```python
from build123d import *

# Parameters (mm, degrees)
SKETCH_1_R               = 4
EXTRUDE_1_DEPTH          = 5.5
SKETCH_2_R               = 1.2
EXTRUDE_2_DEPTH          = 11
SKETCH_6_R               = 0.75
CUT_EXTRUDE_1_DEPTH      = 5
CUT_EXTRUDE_1_DEPTH_BACK = 5
SKETCH_7_R               = 4
CUT_EXTRUDE_2_DEPTH      = 1


with BuildPart() as part:
    # ｽｹｯﾁ1 → ﾎﾞｽ - 押し出し1 (new body)
    with BuildSketch(Plane.XY):
        Circle(SKETCH_1_R)
    extrude(amount=EXTRUDE_1_DEPTH)

    # ｽｹｯﾁ2 → ﾎﾞｽ - 押し出し2 (add)
    with BuildSketch(Plane.XY.offset(5.5)):
        Circle(SKETCH_2_R)
    extrude(amount=EXTRUDE_2_DEPTH)

    # ｽｹｯﾁ4 → ｶｯﾄ - 回転1 (revolve, cut)
    with BuildSketch(Plane(origin=(0, 0, 0), x_dir=(1, 0, 0), z_dir=(0, 1, 0))):
        Polygon((1.2, -16.5), (0.711175277, -16.5), (1.15, -15.5), (0.95, -13.2), (1.2, -12.7), align=None)
    revolve(axis=Axis((0, 0, 12.792952675), (0, 0, 1)), mode=Mode.SUBTRACT)

    # ｽｹｯﾁ6 → ｶｯﾄ - 押し出し1 (cut, two sides)
    with BuildSketch(Plane(origin=(0, 0, 0), x_dir=(1, 0, 0), z_dir=(0, 1, 0))) as cut_extrude_1_sk:
        with Locations((0, -3)):
            Circle(SKETCH_6_R)
    extrude(amount=CUT_EXTRUDE_1_DEPTH, mode=Mode.SUBTRACT)
    extrude(cut_extrude_1_sk.sketch, amount=-CUT_EXTRUDE_1_DEPTH_BACK, mode=Mode.SUBTRACT)

    # ｽｹｯﾁ7 → ｶｯﾄ - 押し出し2 (cut)
    with BuildSketch(Plane(origin=(0, 0, 0), x_dir=(-1, 0, 0), z_dir=(0, 0, -1))):
        Circle(SKETCH_7_R)
    extrude(amount=-CUT_EXTRUDE_2_DEPTH, mode=Mode.SUBTRACT)


solid = part.part
```
Verification items for the finished model (mm, model axes). A direction names the side the tool comes from. Coordinates: 2 decimals unless noted, no trailing zeros. Loops run counter-clockwise (first coordinate to the right, second up) from the corner with the lowest first, then second, coordinate; pieces in that order, holes last. Notation, with made-up numbers: (88.25, 82) -> (143.25, 82) arc R13 cw to (143.25, 107) -> close; hole circle Ø10 at (69, 19). An arc over 180 degrees is marked (long way). Answer in a Markdown table with one row per item. Add a question column.
1. Section check A-A, the plane x = 0. Enter the section's corners in (y, z), then the cut area to 3 significant figures.
2. Access from +Z, -Z, +X, -X, +Y, -Y to the whole of each face (thin tool, end or side, straight path). Record for faces 1 (the face through (0, 0, 1)), 2 (the face through (1, 1, 5.5)), 3 (the face through (-0.227, -1.024, 14.334)).
3. Section check B-B, the plane y = 0. Enter the section's corners in (x, z).
4. Section check D-D, the plane z = 3. Enter the section's corners in (x, y).
5. Material ranges on probe 1 along Z at (x, y) = (0, -0.25); probe 2 along Z at (x, y) = (-3.25, -0.5); probe 3 along Z at (x, y) = (0, -2.25), recorded low to high. Write a range as [from, to].
6. Draft check along Z on faces 4 (the face through (0.65, 1.01, 9.05)), 5 (the face through (0, 0, 16.5)), 6 (the face through (-0.163, 0.056, 3.732)). Enter one of: +Z half, -Z half, draft (parallel to the pull), parting line (faces both ways), or undercut.
7. Section check C-C, the plane z = 8.75. Enter the section's corners in (x, y).
8. Depth check by flat-ended pin: P1, Ø1, axis at x = 0.5, y = -1.5, coming from the +Z side. Enter the tip coordinate at first touch or a pass-through.
Derived:
| question | item | result |
|---|---|---|
| 1 | outline | (-4, 1) -> (4, 1) -> (4, 2.25) -> (-4, 2.25) -> close; (-4, 3.75) -> (4, 3.75) -> (4, 5.5) -> (1.2, 5.5) -> (1.2, 12.7) -> (0.95, 13.2) -> (1.15, 15.5) -> (0.71, 16.5) -> (-0.71, 16.5) -> (-1.15, 15.5) -> (-0.95, 13.2) -> (-1.2, 12.7) -> (-1.2, 5.5) -> (-4, 5.5) -> close |
| 1 | area | 49.0 mm² |
| 2 | face 1 | -Z, +X, -X, +Y, -Y |
| 2 | face 2 | +Z |
| 2 | face 3 | none |
| 3 | outline | (-4, 1) -> (4, 1) -> (4, 5.5) -> (1.2, 5.5) -> (1.2, 12.7) -> (0.95, 13.2) -> (1.15, 15.5) -> (0.71, 16.5) -> (-0.71, 16.5) -> (-1.15, 15.5) -> (-0.95, 13.2) -> (-1.2, 12.7) -> (-1.2, 5.5) -> (-4, 5.5) -> close; hole circle Ø1.5 at (0, 3) |
| 4 | outline | (-0.75, -3.93) -> (-0.75, 3.93) arc R4 ccw to start; (0.75, -3.93) arc R4 ccw to (0.75, 3.93) -> close |
| 5 | probe 1 | z = [1, 2.25], [3.75, 16.5] |
| 5 | probe 2 | z = [1, 5.5] |
| 5 | probe 3 | z = [1, 2.25], [3.75, 5.5] |
| 6 | face 4 | draft |
| 6 | face 5 | +Z half |
| 6 | face 6 | undercut |
| 7 | outline | circle Ø2.4 at (0, 0) |
| 8 | P1 | stops at z = 15.66 |
